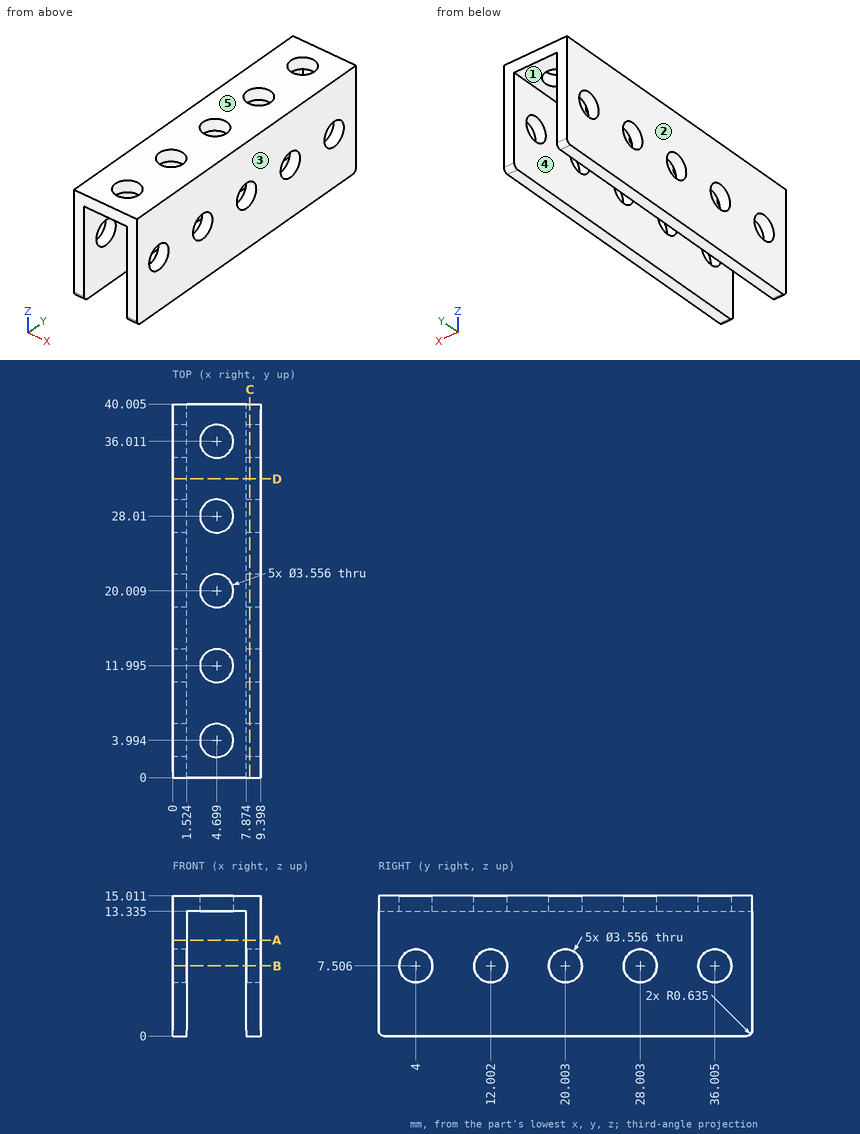
Here's the drawing with two shaded views (mm, measured from the low corner). I have some questions. A direction names the side the tool comes from. Round coordinates to 2 decimals unless told otherwise and drop trailing zeros. Loops run counter-clockwise (first coordinate to the right, second up) from the corner with the lowest first, then second, coordinate; pieces in that order, holes last. Notation, with made-up numbers: M 84.25,3.5 L 136.25,3.5 A24 ccw 136.25,17.5 Z; hole C -21.5,-4.5 d10. An arc over 180 degrees is marked long. Answer as CSV lines item,"result".
1) Which directions (+Z, -Z, +X, -X, +Y, -Y) give clear straight access to the entire face, cutting with the end or side of a thin tool? Please do the marked faces 1 and 2.
From the geometry:
face 1,"-Z, +Y, -Y"
face 2,"+Z, -Z, -X, +Y, -Y"
2) For pin 1 Ø3 at (y, z) = (12, 7.51) entering from +X; pin 2 Ø5.5 at (x, y) = (4.7, 36.01) entering from -Z (1 decimal), each with a flat end and sliding along its axis, tell me the tip position at first contact or that it passes through.
From the geometry:
pin 1,"through"
pin 2,"z = 13.3"
3) Imagine slicing it at A-A on z = 10.25. List the corners of the cut face in (x, y) for me (1 decimal), and give its area (3 significant figures).
From the geometry:
outline,"M 0,0 L 1.5,0 L 1.5,40 L 0,40 Z; M 7.9,0 L 9.4,0 L 9.4,40 L 7.9,40 Z"
area,"122 mm^2"
4) We'd pull the mould along X, two halves only. Please class the marked faces 3, 4 and 5: released by +X, released by -X, zero draft, split by the parting line, or undercut.
From the geometry:
face 3,"released by +X"
face 4,"undercut"
face 5,"zero draft"
5) Imagine slicing it at D-D on y = 32. List the corners of the cut face in (x, z) for me (1 decimal).
From the geometry:
outline,"M 0,0 L 1.5,0 L 1.5,13.3 L 7.9,13.3 L 7.9,0 L 9.4,0 L 9.4,15 L 0,15 Z"
6) Imagine slicing it at C-C on x = 8.25. List the corners of the cut face in (y, z) for me (1 decimal), and give its area (3 significant figures).
From the geometry:
outline,"M 0,0.6 A0.6 ccw 0.6,0 L 39.4,0 A0.6 ccw 40,0.6 L 40,15 L 0,15 Z; hole C 4,7.5 d3.6; hole C 12,7.5 d3.6; hole C 20,7.5 d3.6; hole C 28,7.5 d3.6; hole C 36,7.5 d3.6"
area,"551 mm^2"
7) Imagine slicing it at B-B on z = 7.5. Count the separate pieces of the cut face and the enclosed holes in it.
From the geometry:
separate pieces,"12"
enclosed holes,"0"
8) If I drill on probe 1 along X at (y, z) = (22, 11.5) (1 decimal); probe 2 along Z at (x, y) = (8, 4); probe 3 along Y at (x, z) = (1, 8.75) (1 decimal), over which ranges is the centre line in solid material (lowest first)?
From the geometry:
probe 1,"0 to 1.5, 7.9 to 9.4"
probe 2,"0 to 5.73, 9.28 to 15.01"
probe 3,"0 to 2.7, 5.3 to 10.7, 13.3 to 18.7, 21.3 to 26.7, 29.3 to 34.7, 37.3 to 40"
